Geometry: see drawing. Coordinates: mm, zero at the bounding-box minimum. A direction names the side the tool comes from. Coordinates: 2 decimals unless noted, no trailing zeros. Loops run counter-clockwise (first coordinate to the right, second up) from the corner with the lowest first, then second, coordinate; pieces in that order, holes last. Notation, with made-up numbers: (76.25, -23) - (97.25, -23) arc R35 ccw to (97.25, 15) - close; hole circle Ø5 at (-6.5, -3). An arc over 180 degrees is marked (long way). Use a Markdown table: item, result. Add a question column.
1. Section query A-A on y = 9. Return the cut outline in (x, z) (1 decimal).
2. Section query B-B on z = 30.5. Return the cut outline in (x, y) (1 decimal), then the cut area to 3 significant figures.
3. Contact query for flat-ended pins moving along their axis: P1, Ø10.5, axis at y = 18, z = 9, coming from the -X side; P2, Ø6, axis at x = 12.5, y = 24, coming from the +Z side; P3, Ø6.5, axis at x = 7, z = 7.5, coming from the -Y side; P4, Ø4, axis at x = 20, z = 55.5, coming from the +Y side. Output: stop coordinate, or through.
4. Access query for the marked faces 1, 2 and 3. Directions: +Z, -Z, +X, -X, +Y, -Y. A direction counts if a zero-diameter tool reaches every point of the face in a straight line with its end or side. Return the directions, or none.
5. Ray query, L1, parallel to X at y = 17, z = 55.5 (1 decimal); L2, parallel to Z at x = 1.5, y = 14; L3, parallel to Z at x = 26, y = 29.5. Return the intervals inside material, ascending. Write a range as [from, to].
6. Section query C-C on x = 6. Return the cut outline in (y, z) (1 decimal), then the cut area to 4 significant figures.
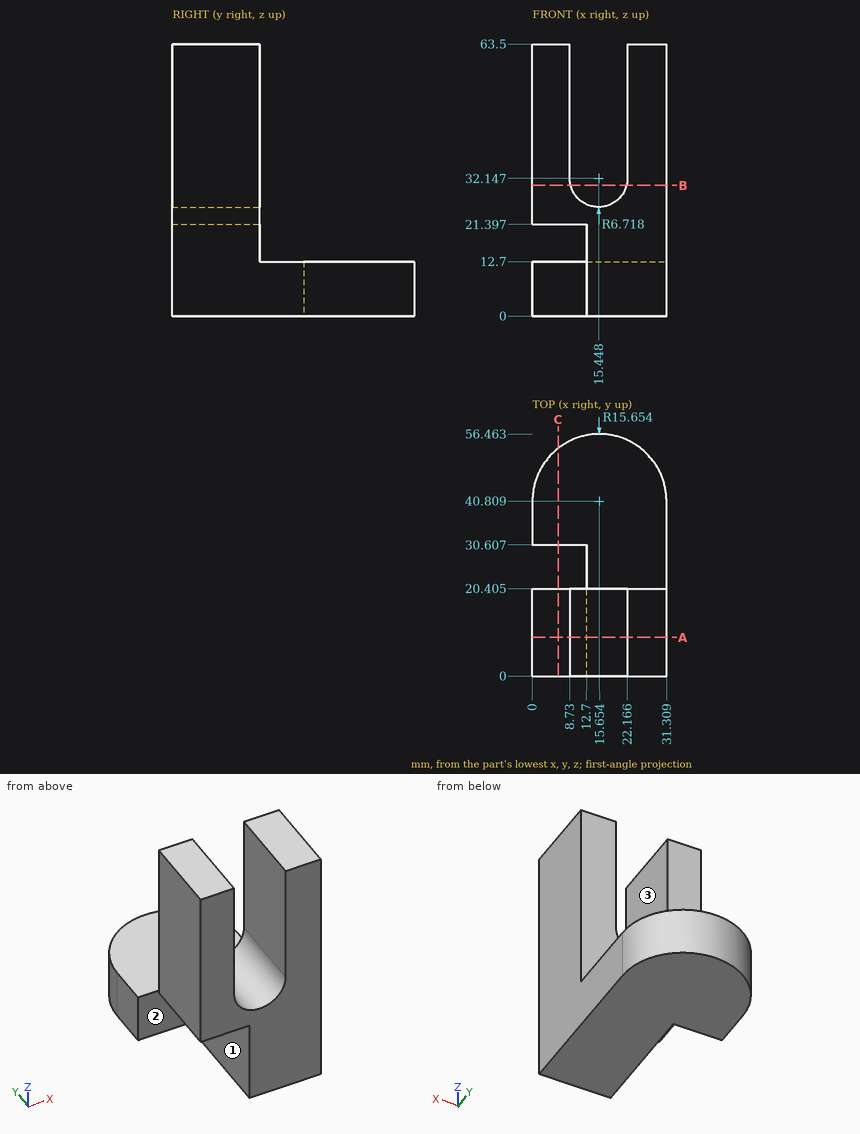
Resolved:
| question | item | result |
|---|---|---|
| 1 | outline | (0, 21.4) - (12.7, 21.4) - (12.7, 0) - (31.3, 0) - (31.3, 63.5) - (22.2, 63.5) - (22.2, 32.1) arc R6.7 cw to (8.7, 32.1) - (8.7, 63.5) - (0, 63.5) - close |
| 2 | outline | (0, 0) - (8.9, 0) - (8.9, 20.4) - (0, 20.4) - close; (22, 0) - (31.3, 0) - (31.3, 20.4) - (22, 20.4) - close |
| 2 | area | 373 mm² |
| 3 | P1 | x = 12.7 |
| 3 | P2 | z = 12.7 |
| 3 | P3 | y = 30.61 |
| 3 | P4 | through |
| 4 | face 1 | -Z, -X, -Y |
| 4 | face 2 | +Z, -Z, -X, -Y |
| 4 | face 3 | +Z, +Y, -Y |
| 5 | L1 | [0, 8.7], [22.2, 31.3] |
| 5 | L2 | [21.4, 63.5] |
| 5 | L3 | [0, 12.7] |
| 6 | outline | (0, 21.4) - (20.4, 21.4) - (20.4, 63.5) - (0, 63.5) - close; (30.6, 0) - (53.1, 0) - (53.1, 12.7) - (30.6, 12.7) - close |
| 6 | area | 1,145 mm² |
